Could you check a few things on this model? Use its own coordinates, in mm. Face numbers are marked on the shaded views. A direction names the side the tool comes from. Coordinates: 2 decimals unless noted, no trailing zeros. Loops run counter-clockwise (first coordinate to the right, second up) from the corner with the lowest first, then second, coordinate; pieces in that order, holes last. Notation, with made-up numbers: (21, 74.25) - (56, 74.25) arc R16 ccw to (56, 92.25) - close; hole circle Ø6 at (56.25, 45). An arc over 180 degrees is marked (long way). One line per question, with ' | ' between items. Start each with the question number.
1. I want a section at A-A, the plane y = -2. Write out the boundary of the cut face in (x, z), then the cut area to 3 significant figures.
2. Please list where these lines run through material, in increasing order: L1, parallel to X at y = -3, z = 17.5; L2, parallel to X at y = 6.75, z = 40; L3, parallel to Y at x = -11.5, z = 47. Write a range as [from, to].
3. We'd pull the mould along X, two halves only. Please class the marked faces 1 and 2: pulls with the +X half, pulls with the -X half, needs draft (parallel to the pull), parting line crosses it, or undercut.
4. I want a section at C-C, the plane y = 5.75. Write out the boundary of the cut face in (x, z).
5. I want a section at B-B, the plane z = 0. Write out the boundary of the cut face in (x, y).
6. I'm going to push flat-ended pins straight in: P1, Ø5, axis at x = 14.5, z = -36, coming from the -Y side; P2, Ø6, axis at y = 4, z = -24, coming from the -X side; P3, Ø3, axis at x = -8.5, y = 2.5, coming from the +Z side. Where does each tip first touch, or does it pass through?
7. Which directions (+Z, -Z, +X, -X, +Y, -Y) give clear straight access to the entire face, cutting with the end or side of a thin tool? Please do the marked faces 3 and 4.
Autodesk Inventor part; units mm, degrees
ref_plane "YZ Plane" through (0, 0, 0) normal (1, 0, 0) x (0, 1, 0)
ref_plane "XZ Plane" through (0, 0, 0) normal (0, 1, 0) x (-1, 0, 0)
ref_plane "XY Plane" through (0, 0, 0) normal (0, 0, 1) x (1, 0, 0)
sketch "Sketch1" plane through (0, 0, 0) normal (0, 1, 0) x (-1, 0, 0)
  circle A0 centre (0, 0) radius 52
  circle A1 centre (0, 0) radius 22.75
  circle A2 centre (0, 0) radius 27.5
  dimension "d2" = 45.5
  dimension "d4" = 55
extrude "Extrusion1" add sketch "Sketch1" against normal blind 4.75 contours A2
extrude "Extrusion2" add sketch "Sketch1" along normal blind 7 contours A0 | A2
fillet "Fillet1" radius 4 1 edges at (52, 0, 0)
sketch "Sketch2" plane through (0, 7, 0) normal (0, 1, 0) x (1, 0, 0)
  circle A0 centre (34.5, 0) radius 10
  circle A1 centre (0, 34.5) radius 10
  circle A2 centre (-34.5, 0) radius 10
  circle A3 centre (0, -34.5) radius 10
  circle A4 centre (0, 0) radius 52
  line L0 (0, 0) -> (44.5, 0)
  circle A5 centre (0, 0) radius 44.5
  dimension "d14" = 360
extrude "Extrusion3" cut sketch "Sketch2" against normal through all contours L0 A0 | A0 L0 | A1 | A2 | A3
sketch "Sketch3" plane through (0, 7, 0) normal (0, 1, 0) x (1, 0, 0)
  circle A0 centre (0, 34.5) radius 10
  arc A1 (6.3329, 26.7609) -> (-6.3329, 26.7609) centre (0, 34.5) ccw
  line L0 (-10, 34.5) -> (-10, 20.4343)
  circle A2 centre (0, 0) radius 22.75
  line L1 (10, 34.5) -> (10, 20.4343)
  line L2 (-34.5, -10) -> (-20.4343, -10)
  line L3 (-34.5, 10) -> (-20.4343, 10)
  line L4 (10, -34.5) -> (10, -20.4343)
  line L5 (-10, -34.5) -> (-10, -20.4343)
  line L6 (34.5, 10) -> (20.4343, 10)
  line L7 (34.5, -10) -> (20.4343, -10)
  circle A3 centre (-34.5, 0) radius 10
  circle A4 centre (34.5, 0) radius 10
  circle A5 centre (0, -34.5) radius 10
  point P0 (-26.7609, 6.3329)
  point P1 (-26.7609, -6.3329)
  point P2 (-6.3329, -26.7609)
  point P3 (6.3329, -26.7609)
  point P4 (34.5, 0)
  point P5 (26.7609, -6.3329)
  point P6 (26.7609, 6.3329)
  point P7 (34.5, 0)
  dimension "d22" = 360
extrude "Extrusion5" cut sketch "Sketch3" against normal through all contours L1 A2 L0 A0 | L6 A4 L7 A2 | A2 L2 A3 L3 | A2 L4 A5 L5
properties part number "wheel_chain_guide_holes"
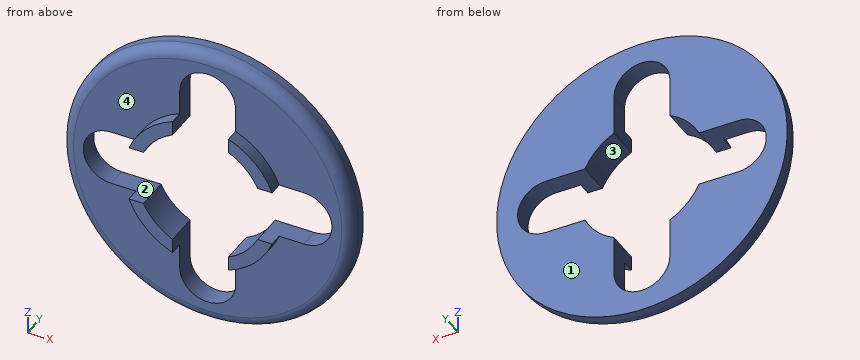
Results are:
1) outline: (-25.62, -10) arc R27.5 ccw to (-10, -25.62) - (-10, -20.43) arc R22.75 cw to (-20.43, -10) - close; (-25.62, 10) - (-20.43, 10) arc R22.75 cw to (-10, 20.43) - (-10, 25.62) arc R27.5 ccw to start; (10, -25.62) arc R27.5 ccw to (25.62, -10) - (20.43, -10) arc R22.75 cw to (10, -20.43) - close; (10, 20.43) arc R22.75 cw to (20.43, 10) - (25.62, 10) arc R27.5 ccw to (10, 25.62) - close | area: 359 mm2
2) L1: x = [-21.21, -14.54], [14.54, 21.21] | L2: x = [-33.23, -8.35], [8.35, 33.23] | L3: y = [0.02, 7]
3) face 1: needs draft | face 2: undercut
4) outline: circle Ø104 at (0, 0); hole (-34.5, -10) - (-20.43, -10) arc R22.75 ccw to (-10, -20.43) - (-10, -34.5) arc R10 ccw to (10, -34.5) - (10, -20.43) arc R22.75 ccw to (20.43, -10) - (34.5, -10) arc R10 ccw to (34.5, 10) - (20.43, 10) arc R22.75 ccw to (10, 20.43) - (10, 34.5) arc R10 ccw to (-10, 34.5) - (-10, 20.43) arc R22.75 ccw to (-20.43, 10) - (-34.5, 10) arc R10 ccw to start
5) outline: (-52, 4) arc R4 ccw to (-48, 0) - (-44.5, 0) - (-44.5, 7) - (-52, 7) - close; (44.5, 0) - (48, 0) arc R4 ccw to (52, 4) - (52, 7) - (44.5, 7) - close
6) P1: stops at y = 0 | P2: stops at x = -47.57 | P3: stops at z = 51.44
7) face 3: +Y, -Y | face 4: -Y
